Autodesk Inventor part; units mm, degrees
ref_plane "YZ Plane" through (0, 0, 0) normal (1, 0, 0) x (0, 1, 0)
ref_plane "XZ Plane" through (0, 0, 0) normal (0, 1, 0) x (-1, 0, 0)
ref_plane "XY Plane" through (0, 0, 0) normal (0, 0, 1) x (1, 0, 0)
sketch "Sketch1" plane through (0, 0, 0) normal (0, 0, 1) x (1, 0, 0)
  line L0 (3.9874, -107.95) -> (-5.3154, -107.95) construction
  line L1 (6.3686, -83.7157) -> (6.3686, -107.95) construction
  line L2 (6.3686, -107.95) -> (-38.0814, -107.95)
  line L3 (-44.4314, -82.55) -> (-44.4314, 82.55)
  line L4 (-38.0814, 107.95) -> (6.3686, 107.95)
  line L5 (6.3686, 107.95) -> (6.3686, -107.95)
  line L6 (-44.4314, -107.95) -> (-38.0814, -107.95) construction
  line L7 (-44.4314, -107.95) -> (-44.4314, -82.55) construction
  line L8 (-44.4314, 107.95) -> (-38.0814, 107.95) construction
  line L9 (-44.4314, 107.95) -> (-44.4314, 82.55) construction
  line L10 (-38.0814, 107.95) -> (-44.4314, 82.55)
  line L11 (-44.4314, -82.55) -> (-38.0814, -107.95)
  line L12 (-44.4314, 107.95) -> (-44.4314, 101.6) construction
  line L13 (-44.4314, 107.95) -> (-31.7314, 107.95) construction
  line L14 (-44.4314, -107.95) -> (-31.7314, -107.95) construction
  line L15 (-44.4314, -107.95) -> (-44.4314, -101.6) construction
  circle A0 centre (-31.7314, -101.6) radius 2.1844
  circle A1 centre (-31.7314, 101.6) radius 2.1844
  point P0 (0, 0)
  dimension "d0" = 50.8
  dimension "d1" = 215.9
  dimension "d2" = 6.35
  dimension "d3" = 25.4
  dimension "d4" = 6.35
  dimension "d5" = 25.4
  dimension "d8" = 6.35
  dimension "d9" = 12.7
  dimension "d10" = 12.7
  dimension "d11" = 6.35
  dimension "d12" = 4.3688
  dimension "d13" = 4.3688
extrude "Extrusion1" add sketch "Sketch1" along normal blind 1.5875
properties part number "Angle changer polycarb"
Could you check a few things on this model? Use its own coordinates, in mm. Give positions to 0.01 mm unless a question says otherwise; leave off trailing zeros. Order: outer loops, then holes, each group sorted by start corner. A loop starts at its lowest first (then second) coordinate and runs counter-clockwise, first axis right, second up. Notation, with made-up numbers: (43.5, 2.25) - (87.5, 2.25) arc R20 ccw to (87.5, 24.25) - close; hole circle Ø3 at (44.25, -18). An arc over 180 degrees is marked (long way). Return JSON: item names as keys, results as strings. Group by question number.
Q1. Thinking about a two-plate mould opening in X: for faces 1 (the face through (-41.3, -95.07, 0.78)), 2 (the face through (-32.205, 103.732, 0.783)), 3 (the face through (-19, 2, 1.588)), 4 (the face through (-32.205, -99.468, 0.783)), which applies, pulls with the +X half, pulls with the -X half, needs draft (parallel to the pull), parting line crosses it, or undercut?
Q2. Please list where these lines run through material, in increasing order: line 1 along X through (y, z) = (-88, 1.15); line 2 along X through (y, z) = (84, 0.9). Write a range as [from, to].
Q3. Will this pin go through, and if not, where does the flat tip stop? pin 1 Ø3.5 at (x, y) = (-31.73, -101.6) entering from +Z.
Q4. Suppose I cut it at B-B, the plane y = -101.6. Please give me the cut outline in (x, z), and give its area (3 significant figures).
Q5. Suppose I cut it at A-A, the plane z = 0.9. Please give me the cut outline in (x, y).
Resolved:
{
 "1": {"face 1": "pulls with the -X half", "face 2": "undercut", "face 3": "needs draft", "face 4": "undercut"},
 "2": {"line 1": "x = [-43.07, 6.37]", "line 2": "x = [-44.07, 6.37]"},
 "3": {"pin 1": "passes through"},
 "4": {"outline": "(-39.67, 0) - (-33.92, 0) - (-33.92, 1.59) - (-39.67, 1.59) - close; (-29.55, 0) - (6.37, 0) - (6.37, 1.59) - (-29.55, 1.59) - close", "area": "66.1 mm2"},
 "5": {"outline": "(-44.43, -82.55) - (-38.08, -107.95) - (6.37, -107.95) - (6.37, 107.95) - (-38.08, 107.95) - (-44.43, 82.55) - close; hole circle Ø4.37 at (-31.73, -101.6); hole circle Ø4.37 at (-31.73, 101.6)"}
}
